from build123d import *

# Parameters (mm, degrees)
MODEL_R             = 3.05
MODEL_R_2           = 1.75
BOSS_EXTRUDE2_DEPTH = 8


with BuildPart() as part:
    # Model → Boss-Extrude2 (new body)
    with BuildSketch(Plane.XY):
        with BuildLine():
            Line((-92.5, 21.8), (-92.5, 2))
            Line((-92.5, 2), (-92.5, 0))
            Line((-92.5, 0), (-90.5, 0))
            Line((-90.5, 0), (90.5, 0))
            Line((90.5, 0), (92.5, 0))
            Line((92.5, 0), (92.5, 2))
            Line((92.5, 2), (92.5, 21.8))
            ThreePointArc((92.5, 21.8), (92.441421356, 21.941421356), (92.3, 22))
            Line((92.3, 22), (78.7, 22))
            ThreePointArc((78.7, 22), (78.558578644, 21.941421356), (78.5, 21.8))
            Line((78.5, 21.8), (78.5, 20.2))
            ThreePointArc((78.5, 20.2), (78.441421356, 20.058578644), (78.3, 20))
            Line((78.3, 20), (73.5, 20))
            ThreePointArc((73.5, 20), (73.358578644, 20.058578644), (73.3, 20.2))
            Line((73.3, 20.2), (73.3, 21.8))
            ThreePointArc((73.3, 21.8), (73.241421356, 21.941421356), (73.1, 22))
            Line((73.1, 22), (67.3, 22))
            ThreePointArc((67.3, 22), (65.885786438, 22.585786438), (65.3, 24))
            Line((65.3, 24), (65.3, 26))
            ThreePointArc((65.3, 26), (65.885786438, 27.414213562), (67.3, 28))
            Line((67.3, 28), (73.1, 28))
            ThreePointArc((73.1, 28), (73.241421356, 28.058578644), (73.3, 28.2))
            Line((73.3, 28.2), (73.3, 29.8))
            ThreePointArc((73.3, 29.8), (73.358578644, 29.941421356), (73.5, 30))
            Line((73.5, 30), (78.3, 30))
            ThreePointArc((78.3, 30), (78.441421356, 29.941421356), (78.5, 29.8))
            Line((78.5, 29.8), (78.5, 28.2))
            ThreePointArc((78.5, 28.2), (78.558578644, 28.058578644), (78.7, 28))
            Line((78.7, 28), (92.3, 28))
            ThreePointArc((92.3, 28), (92.441421356, 28.058578644), (92.5, 28.2))
            Line((92.5, 28.2), (92.5, 36.25))
            Line((92.5, 36.25), (100.5, 36.25))
            Line((100.5, 36.25), (100.5, 56.25))
            Line((100.5, 56.25), (92.5, 56.25))
            Line((92.5, 56.25), (92.5, 78.75))
            Line((92.5, 78.75), (100.5, 78.75))
            Line((100.5, 78.75), (100.5, 98.75))
            Line((100.5, 98.75), (92.5, 98.75))
            Line((92.5, 98.75), (92.5, 106.8))
            ThreePointArc((92.5, 106.8), (92.441421356, 106.941421356), (92.3, 107))
            Line((92.3, 107), (78.7, 107))
            ThreePointArc((78.7, 107), (78.558578644, 106.941421356), (78.5, 106.8))
            Line((78.5, 106.8), (78.5, 105.2))
            ThreePointArc((78.5, 105.2), (78.441421356, 105.058578644), (78.3, 105))
            Line((78.3, 105), (73.5, 105))
            ThreePointArc((73.5, 105), (73.358578644, 105.058578644), (73.3, 105.2))
            Line((73.3, 105.2), (73.3, 106.8))
            ThreePointArc((73.3, 106.8), (73.241421356, 106.941421356), (73.1, 107))
            Line((73.1, 107), (67.3, 107))
            ThreePointArc((67.3, 107), (65.885786438, 107.585786438), (65.3, 109))
            Line((65.3, 109), (65.3, 111))
            ThreePointArc((65.3, 111), (65.885786438, 112.414213562), (67.3, 113))
            Line((67.3, 113), (73.1, 113))
            ThreePointArc((73.1, 113), (73.241421356, 113.058578644), (73.3, 113.2))
            Line((73.3, 113.2), (73.3, 114.8))
            ThreePointArc((73.3, 114.8), (73.358578644, 114.941421356), (73.5, 115))
            Line((73.5, 115), (78.3, 115))
            ThreePointArc((78.3, 115), (78.441421356, 114.941421356), (78.5, 114.8))
            Line((78.5, 114.8), (78.5, 113.2))
            ThreePointArc((78.5, 113.2), (78.558578644, 113.058578644), (78.7, 113))
            Line((78.7, 113), (92.3, 113))
            ThreePointArc((92.3, 113), (92.441421356, 113.058578644), (92.5, 113.2))
            Line((92.5, 113.2), (92.5, 133))
            Line((92.5, 133), (92.5, 135))
            Line((92.5, 135), (90.5, 135))
            Line((90.5, 135), (14.5, 135))
            Line((14.5, 135), (14.5, 25))
            Line((14.5, 25), (-24.5, 25))
            Line((-24.5, 25), (-24.5, 135))
            Line((-24.5, 135), (-90.5, 135))
            Line((-90.5, 135), (-92.5, 135))
            Line((-92.5, 135), (-92.5, 133))
            Line((-92.5, 133), (-92.5, 113.2))
            ThreePointArc((-92.5, 113.2), (-92.441421356, 113.058578644), (-92.3, 113))
            Line((-92.3, 113), (-78.7, 113))
            ThreePointArc((-78.7, 113), (-78.558578644, 113.058578644), (-78.5, 113.2))
            Line((-78.5, 113.2), (-78.5, 114.8))
            ThreePointArc((-78.5, 114.8), (-78.441421356, 114.941421356), (-78.3, 115))
            Line((-78.3, 115), (-73.5, 115))
            ThreePointArc((-73.5, 115), (-73.358578644, 114.941421356), (-73.3, 114.8))
            Line((-73.3, 114.8), (-73.3, 113.2))
            ThreePointArc((-73.3, 113.2), (-73.241421356, 113.058578644), (-73.1, 113))
            Line((-73.1, 113), (-67.3, 113))
            ThreePointArc((-67.3, 113), (-65.885786438, 112.414213562), (-65.3, 111))
            Line((-65.3, 111), (-65.3, 109))
            ThreePointArc((-65.3, 109), (-65.885786438, 107.585786438), (-67.3, 107))
            Line((-67.3, 107), (-73.1, 107))
            ThreePointArc((-73.1, 107), (-73.241421356, 106.941421356), (-73.3, 106.8))
            Line((-73.3, 106.8), (-73.3, 105.2))
            ThreePointArc((-73.3, 105.2), (-73.358578644, 105.058578644), (-73.5, 105))
            Line((-73.5, 105), (-78.3, 105))
            ThreePointArc((-78.3, 105), (-78.441421356, 105.058578644), (-78.5, 105.2))
            Line((-78.5, 105.2), (-78.5, 106.8))
            ThreePointArc((-78.5, 106.8), (-78.558578644, 106.941421356), (-78.7, 107))
            Line((-78.7, 107), (-92.3, 107))
            ThreePointArc((-92.3, 107), (-92.441421356, 106.941421356), (-92.5, 106.8))
            Line((-92.5, 106.8), (-92.5, 98.75))
            Line((-92.5, 98.75), (-100.5, 98.75))
            Line((-100.5, 98.75), (-100.5, 78.75))
            Line((-100.5, 78.75), (-92.5, 78.75))
            Line((-92.5, 78.75), (-92.5, 56.25))
            Line((-92.5, 56.25), (-100.5, 56.25))
            Line((-100.5, 56.25), (-100.5, 36.25))
            Line((-100.5, 36.25), (-92.5, 36.25))
            Line((-92.5, 36.25), (-92.5, 28.2))
            ThreePointArc((-92.5, 28.2), (-92.441421356, 28.058578644), (-92.3, 28))
            Line((-92.3, 28), (-78.7, 28))
            ThreePointArc((-78.7, 28), (-78.558578644, 28.058578644), (-78.5, 28.2))
            Line((-78.5, 28.2), (-78.5, 29.8))
            ThreePointArc((-78.5, 29.8), (-78.441421356, 29.941421356), (-78.3, 30))
            Line((-78.3, 30), (-73.5, 30))
            ThreePointArc((-73.5, 30), (-73.358578644, 29.941421356), (-73.3, 29.8))
            Line((-73.3, 29.8), (-73.3, 28.2))
            ThreePointArc((-73.3, 28.2), (-73.241421356, 28.058578644), (-73.1, 28))
            Line((-73.1, 28), (-67.3, 28))
            ThreePointArc((-67.3, 28), (-65.885786438, 27.414213562), (-65.3, 26))
            Line((-65.3, 26), (-65.3, 24))
            ThreePointArc((-65.3, 24), (-65.885786438, 22.585786438), (-67.3, 22))
            Line((-67.3, 22), (-73.1, 22))
            ThreePointArc((-73.1, 22), (-73.241421356, 21.941421356), (-73.3, 21.8))
            Line((-73.3, 21.8), (-73.3, 20.2))
            ThreePointArc((-73.3, 20.2), (-73.358578644, 20.058578644), (-73.5, 20))
            Line((-73.5, 20), (-78.3, 20))
            ThreePointArc((-78.3, 20), (-78.441421356, 20.058578644), (-78.5, 20.2))
            Line((-78.5, 20.2), (-78.5, 21.8))
            ThreePointArc((-78.5, 21.8), (-78.558578644, 21.941421356), (-78.7, 22))
            Line((-78.7, 22), (-92.3, 22))
            ThreePointArc((-92.3, 22), (-92.441421356, 21.941421356), (-92.5, 21.8))
        make_face()
        with Locations(Location((-32, 55, 0), (0, 0, 180))):
            Circle(MODEL_R, mode=Mode.SUBTRACT)
        with Locations((-32, 70)):
            Circle(MODEL_R, mode=Mode.SUBTRACT)
        with Locations(Location((22, 100, 0), (0, 0, 180))):
            Circle(MODEL_R, mode=Mode.SUBTRACT)
        with Locations((22, 85)):
            Circle(MODEL_R, mode=Mode.SUBTRACT)
        with Locations((22, 25)):
            Circle(MODEL_R, mode=Mode.SUBTRACT)
        with Locations(Location((22, 40, 0), (0, 0, 180))):
            Circle(MODEL_R, mode=Mode.SUBTRACT)
        with Locations((-32, 40)):
            Circle(MODEL_R, mode=Mode.SUBTRACT)
        with Locations(Location((-32, 25, 0), (0, 0, 180))):
            Circle(MODEL_R, mode=Mode.SUBTRACT)
        with Locations(Location((22, 70, 0), (0, 0, 180))):
            Circle(MODEL_R, mode=Mode.SUBTRACT)
        with Locations((22, 55)):
            Circle(MODEL_R, mode=Mode.SUBTRACT)
        with Locations((22, 115)):
            Circle(MODEL_R, mode=Mode.SUBTRACT)
        with Locations(Location((-32, 115, 0), (0, 0, 180))):
            Circle(MODEL_R, mode=Mode.SUBTRACT)
        with Locations(Location((-32, 85, 0), (0, 0, 180))):
            Circle(MODEL_R, mode=Mode.SUBTRACT)
        with Locations((-32, 100)):
            Circle(MODEL_R, mode=Mode.SUBTRACT)
        with Locations((-5, 15)):
            Circle(MODEL_R_2, mode=Mode.SUBTRACT)
    extrude(amount=BOSS_EXTRUDE2_DEPTH)


solid = part.part
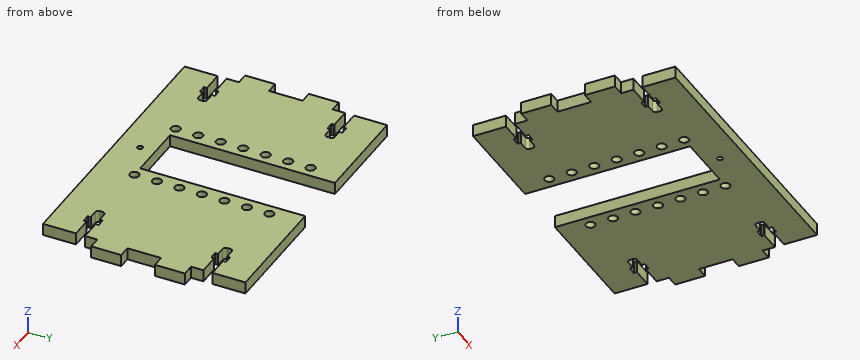
Could you check a few things on this model? Use its own coordinates, in mm. Round coordinates to 2 decimals unless told otherwise and drop trailing zeros. Write each loop counter-clockwise with the first axis right and the second up, starting at its lowest first coordinate (ties: lowest second). Pieces come first, ordered by that corner, then holes. Notation, with made-up numbers: (64, 15.25) - (107, 15.25) arc R26 ccw to (107, 30.25) - close; hole circle Ø5 at (-16.5, -4). An arc over 180 degrees is marked (long way). Use a Markdown table: item, result.
Q1. For pin 1 (2.5 mm diameter, centred on x = 96, z = 2.5, fed in from +Y); pin 2 (0.6 mm diameter, centred on y = 109.5, z = 5.5, fed in from +X); pin 3 (4 mm diameter, centred on x = 97, z = 4, fed in from -Y); pin 4 (5.5 mm diameter, centred on x = -32, y = 70, fed in from -Z), each with a flat end and sliding along its axis, tell me the tip position at first contact or that it passes through.
Output values:
| item | result |
|---|---|
| pin 1 | y = 98.75 |
| pin 2 | x = 65.3 |
| pin 3 | y = 36.25 |
| pin 4 | through |
Q2. I want a section at B-B (y = 85). List the corners of the cut face in (x, z) for me, plus the area to 3 significant figures.
Output values:
| item | result |
|---|---|
| outline | (-100.5, 0) - (-35.05, 0) - (-35.05, 8) - (-100.5, 8) - close; (-28.95, 0) - (-24.5, 0) - (-24.5, 8) - (-28.95, 8) - close; (14.5, 0) - (18.95, 0) - (18.95, 8) - (14.5, 8) - close; (25.05, 0) - (100.5, 0) - (100.5, 8) - (25.05, 8) - close |
| area | 1,200 mm2 |
Q3. I want a section at A-A (x = 22). Count the separate pieces of the cut face and the enclosed holes in it, plus the area to 3 significant figures.
Output values:
| item | result |
|---|---|
| separate pieces | 8 |
| enclosed holes | 0 |
| area | 738 mm2 |
Q4. I want a section at C-C (x = 87). List the corners of the cut face in (y, z) for me, plus the area to 3 significant figures.
Output values:
| item | result |
|---|---|
| outline | (0, 0) - (22, 0) - (22, 8) - (0, 8) - close; (28, 0) - (107, 0) - (107, 8) - (28, 8) - close; (113, 0) - (135, 0) - (135, 8) - (113, 8) - close |
| area | 984 mm2 |
Q5. I want a section at D-D (y = 70). List the corners of the cut face in (x, z) for me.
Output values:
| item | result |
|---|---|
| outline | (-92.5, 0) - (-35.05, 0) - (-35.05, 8) - (-92.5, 8) - close; (-28.95, 0) - (-24.5, 0) - (-24.5, 8) - (-28.95, 8) - close; (14.5, 0) - (18.95, 0) - (18.95, 8) - (14.5, 8) - close; (25.05, 0) - (92.5, 0) - (92.5, 8) - (25.05, 8) - close |
Q6. Please list where these lines run through material, in increasing order: L1, parallel to X at y = 31, z = 7.5; L2, parallel to Y at x = 8.5, z = 1.5; L3, parallel to X at y = 50.5, z = 3.25.
Output values:
| item | result |
|---|---|
| L1 | -92.5 to -24.5, 14.5 to 92.5 |
| L2 | 0 to 25 |
| L3 | -100.5 to -24.5, 14.5 to 100.5 |
